Input: part model. Units: mm. Frame: model coordinates. Face numbers are marked on the shaded views. A direction names the side the tool comes from. Round coordinates to 2 decimals unless told otherwise and drop trailing zeros. Order: outer loops, then holes, each group sorted by start corner. A loop starts at its lowest first (then second) coordinate and runs counter-clockwise, first axis right, second up. Notation, with made-up numbers: (75, 26.5) -> (109, 26.5) arc R11 cw to (109, 45.5) -> close; hole circle Ø1 at (-14.75, 33). An arc over 180 degrees is marked (long way). Use a Markdown table: item, result.
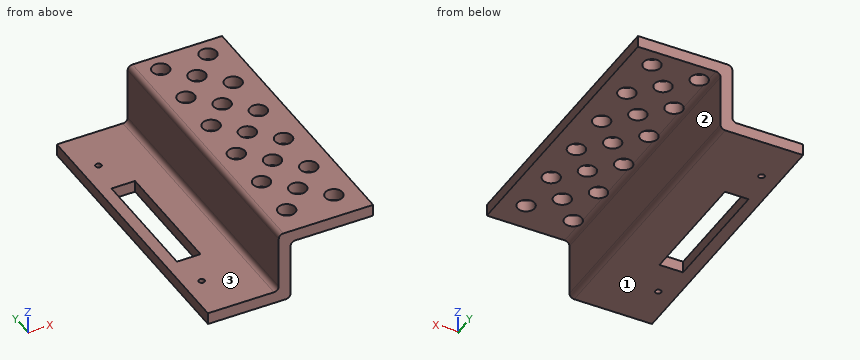
from build123d import *

# Parameters (mm, degrees)
F1_DEPTH = 76.2
F2_R     = 0.79375
F2_W     = 6.35
F2_H     = 33.02
F3_DEPTH = 5.842
F4_R     = 2.3114
F5_DEPTH = 3.81


with BuildPart() as f1:
    # F0 (on Front) → F1 (new body)
    with BuildSketch(Plane.XZ):
        with BuildLine():
            Line((-29.730175, 55.896019), (-53.860175, 55.896019))
            ThreePointArc((-53.860175, 55.896019), (-54.7582, 55.524044), (-55.130175, 54.626019))
            Line((-55.130175, 54.626019), (-55.130175, 52.721019))
            Line((-55.130175, 52.721019), (-55.130175, 40.656019))
            ThreePointArc((-55.130175, 40.656019), (-55.502149, 39.757993), (-56.400175, 39.386019))
            Line((-56.400175, 39.386019), (-74.180175, 39.386019))
            Line((-74.180175, 39.386019), (-74.180175, 36.211019))
            Line((-74.180175, 36.211019), (-55.130175, 36.211019))
            Line((-55.130175, 36.211019), (-53.225175, 36.211019))
            ThreePointArc((-53.225175, 36.211019), (-52.327149, 36.582993), (-51.955175, 37.481019))
            Line((-51.955175, 37.481019), (-51.955175, 51.451019))
            ThreePointArc((-51.955175, 51.451019), (-51.5832, 52.349044), (-50.685175, 52.721019))
            Line((-50.685175, 52.721019), (-29.730175, 52.721019))
            Line((-29.730175, 52.721019), (-29.730175, 55.896019))
        make_face()
    extrude(amount=F1_DEPTH)

    # F2 (on face) → F3 (cut)
    with BuildSketch(Plane.XY.offset(39.386019)):
        with Locations((-69.417675, -64.135)):
            Circle(F2_R)
        with Locations((-67.830175, -38.1)):
            Rectangle(F2_W, F2_H)
        with Locations((-69.417675, -12.065)):
            Circle(F2_R)
    extrude(amount=-F3_DEPTH, mode=Mode.SUBTRACT)

    # F4 (on face) → F5 (cut)
    with BuildSketch(Plane.XY.offset(55.896019)):
        with Locations((-48.780175, -55.608343)):
            Circle(F4_R)
        with Locations((-48.780175, -68.308343)):
            Circle(F4_R)
        with Locations((-42.430175, -61.958343)):
            Circle(F4_R)
        with Locations((-36.080175, -68.308343)):
            Circle(F4_R)
        with Locations((-36.080175, -55.608343)):
            Circle(F4_R)
        with Locations((-36.080175, -42.908343)):
            Circle(F4_R)
        with Locations((-42.430175, -49.258343)):
            Circle(F4_R)
        with Locations((-48.780175, -42.908343)):
            Circle(F4_R)
        with Locations((-42.430175, -36.558343)):
            Circle(F4_R)
        with Locations((-36.080175, -30.208343)):
            Circle(F4_R)
        with Locations((-48.780175, -30.208343)):
            Circle(F4_R)
        with Locations((-42.430175, -23.858343)):
            Circle(F4_R)
        with Locations((-36.080175, -17.508343)):
            Circle(F4_R)
        with Locations((-42.430175, -11.158343)):
            Circle(F4_R)
        with Locations((-48.780175, -17.508343)):
            Circle(F4_R)
        with Locations((-36.080175, -4.808343)):
            Circle(F4_R)
        with Locations((-48.780175, -4.808343)):
            Circle(F4_R)
    extrude(amount=-F5_DEPTH, mode=Mode.SUBTRACT)


solid = f1.part
1) Cut plane C-C on z = 50.5. Return loops of the section in (x, y), and give its area (3 significant figures).
Answer key:
| item | result |
|---|---|
| outline | (-55.13, -76.2) -> (-51.96, -76.2) -> (-51.96, 0) -> (-55.13, 0) -> close |
| area | 242 mm^2 |
2) Cut plane B-B on y = -8. Return loops of the section in (x, z), and give its area (3 significant figures).
Answer key:
| item | result |
|---|---|
| outline | (-74.18, 36.21) -> (-53.23, 36.21) arc R1.27 ccw to (-51.96, 37.48) -> (-51.96, 51.45) arc R1.27 cw to (-50.69, 52.72) -> (-29.73, 52.72) -> (-29.73, 55.9) -> (-53.86, 55.9) arc R1.27 ccw to (-55.13, 54.63) -> (-55.13, 40.66) arc R1.27 cw to (-56.4, 39.39) -> (-74.18, 39.39) -> close |
| area | 194 mm^2 |
3) Cut plane A-A on x = -37. Return loops of the section in (y, z).
Answer key:
| item | result |
|---|---|
| outline | (-76.2, 52.72) -> (-70.43, 52.72) -> (-70.43, 55.9) -> (-76.2, 55.9) -> close; (-66.19, 52.72) -> (-57.73, 52.72) -> (-57.73, 55.9) -> (-66.19, 55.9) -> close; (-53.49, 52.72) -> (-45.03, 52.72) -> (-45.03, 55.9) -> (-53.49, 55.9) -> close; (-40.79, 52.72) -> (-32.33, 52.72) -> (-32.33, 55.9) -> (-40.79, 55.9) -> close; (-28.09, 52.72) -> (-19.63, 52.72) -> (-19.63, 55.9) -> (-28.09, 55.9) -> close; (-15.39, 52.72) -> (-6.93, 52.72) -> (-6.93, 55.9) -> (-15.39, 55.9) -> close; (-2.69, 52.72) -> (0, 52.72) -> (0, 55.9) -> (-2.69, 55.9) -> close |
4) Set-up query: the marked faces 1, 2 and 3. Return all of +Z, -Z, +X, -X, +Y, -Y with unobstructed straight access to the full face (end or side cutting, diameter ignored); none if empty.
Answer key:
| item | result |
|---|---|
| face 1 | -Z, +X, -X, +Y, -Y |
| face 2 | -Z, +X, +Y, -Y |
| face 3 | +Z, -X, +Y, -Y |
5) Contact query for flat-ended pins moving along their axis: P1, Ø6, axis at y = -18, z = 51, coming from the -X side; P2, Ø7.5, axis at x = -42.43, y = -23.86, coming from the +Z side; P3, Ø5.5, axis at x = -36.08, y = -30.21, coming from the -Z side; P4, Ø6, axis at y = -8, z = 43, coming from the +X side. Output: stop coordinate, or through.
Answer key:
| item | result |
|---|---|
| P1 | stops at x = -55.13 |
| P2 | stops at z = 55.9 |
| P3 | stops at z = 52.72 |
| P4 | stops at x = -51.96 |
6) Ray query, probe 1 along Z at (x, y) = (-69, -20); probe 2 along Y at (x, z) = (-70, 37.25); probe 3 along X at (y, z) = (-66.5, 38). Return the intervals inside material, ascending.
Answer key:
| item | result |
|---|---|
| probe 1 | z = 36.21 to 39.39 |
| probe 2 | y = -76.2 to -64.67, -63.6 to -54.61, -21.59 to -12.6, -11.53 to 0 |
| probe 3 | x = -74.18 to -51.96 |
